For this review, take the finished solid that the model builds, in its own axes (mm). A direction names the side the tool comes from. Coordinates: 2 decimals unless noted, no trailing zeros. Write each loop counter-clockwise with the first axis right and the second up, starting at its lowest first coordinate (ties: lowest second). Pieces come first, ordered by that corner, then holes. Notation, with made-up numbers: (84, 40) -> (142, 40) arc R18 cw to (142, 72) -> close; hole circle Ø10 at (21.25, 21.5). An arc over 180 degrees is marked (long way). One line per item, written item: value. Start each with the question number.
1) Add section A-A (y = 50). State the section outline as (x, z) points, and give its area (3 significant figures).
2) For probe 1 along Y at (x, z) = (53, 51.5); probe 2 along X at (y, z) = (39, 12.5); probe 3 along Z at (x, y) = (0.95, -50), list the stretches that pass through material, from the lowest coordinate up. Write a range as from..to.
3) Add section B-B (z = 35). State the section outline as (x, y) points.
4) Add section D-D (x = 13). State the section outline as (y, z) points, and give its area (4 significant figures).
5) Add section C-C (y = 27). State the section outline as (x, z) points, and give its area (3 significant figures).
6) Mouldability with a two-part tool opening along Z and no side actions: class faces 1 (the flat face through (30, 63.5, 39)), 2 (the flat face through (35, 1, 0)), 3 (the cylindrical face through (0.7, -49.6, 3.4)) as released by +Z, released by -Z, zero draft, split by the parting line, or undercut.
7) For pin 1 Ø22.5 at (x, y) = (34, 48) entering from +Z; pin 2 Ø3 at (y, z) = (-8.5, 73.39) entering from -X, all flat-tipped, find the tip position at first contact; note any pin that passes through.
8) Machinability: for faces 4 (the cylindrical face through (0.74, -24.12, 63.17)), 5 (the flat face through (31, -62, 40)), 6 (the flat face through (1, 0, 80)), which of the approach directions +Z, -Z, +X, -X, +Y, -Y give a long, thin tool a straight path to every point of the face, cutting with its end or side? Answer none if there is none.
from build123d import *

# Parameters (mm, degrees)
PAD_DEPTH       = 80
POCKET_DEPTH    = 79.001
SKETCH002_R     = 1.65
POCKET001_DEPTH = 5


with BuildPart() as part:
    # Sketch → Pad (new body)
    with BuildSketch(Plane.XY):
        with BuildLine():
            Line((0, 63.5), (60, 63.5))
            ThreePointArc((70, 53.5), (67.071068, 60.571068), (60, 63.5))
            Line((70, 53.5), (70, -53.5))
            ThreePointArc((60, -63.5), (67.071068, -60.571068), (70, -53.5))
            Line((60, -63.5), (0, -63.5))
            Line((0, -63.5), (0, 63.5))
        make_face()
    extrude(amount=PAD_DEPTH)

    # Sketch001 → Pocket (cut, through all)
    with BuildSketch(Plane.XY.offset(1)):
        with BuildLine():
            Line((1.5, 62), (60, 62))
            ThreePointArc((68.5, 53.5), (66.010408, 59.510408), (60, 62))
            Line((68.5, 53.5), (68.5, 17))
            Line((68.5, 17), (1.5, 17))
            Line((1.5, 17), (1.5, 62))
        make_face()
        with BuildLine():
            Line((1.5, 15.5), (68.5, 15.5))
            Line((68.5, 15.5), (68.5, -53.5))
            ThreePointArc((60, -62), (66.010408, -59.510408), (68.5, -53.5))
            Line((60, -62), (1.5, -62))
            Line((1.5, -62), (1.5, 15.5))
        make_face()
    extrude(amount=POCKET_DEPTH, mode=Mode.SUBTRACT)

    # Sketch002 → Pocket001 (cut)
    with BuildSketch(Plane(origin=(0, 0, 0), x_dir=(0, -1, 0), z_dir=(-1, 0, 0))):
        with Locations((-50, 5)):
            Circle(SKETCH002_R)
        with Locations((50, 5)):
            Circle(SKETCH002_R)
        with Locations((8.5, 73.394079)):
            Circle(SKETCH002_R)
        with Locations((24.47625, 64.779078)):
            Circle(SKETCH002_R)
    extrude(amount=-POCKET001_DEPTH, mode=Mode.SUBTRACT)


solid = part.part
Numbers:
1. outline: (0, 0) -> (70, 0) -> (70, 80) -> (68.5, 80) -> (68.5, 1) -> (1.5, 1) -> (1.5, 3.35) -> (0, 3.35) -> close; (0, 6.65) -> (1.5, 6.65) -> (1.5, 80) -> (0, 80) -> close
1. area: 302 mm²
2. probe 1: -63.5..-62, 15.5..17, 62..63.5
2. probe 2: 0..1.5, 68.5..70
2. probe 3: 0..3.35, 6.65..80
3. outline: (0, -63.5) -> (60, -63.5) arc R10 ccw to (70, -53.5) -> (70, 53.5) arc R10 ccw to (60, 63.5) -> (0, 63.5) -> close; hole (1.5, -62) -> (60, -62) arc R8.5 ccw to (68.5, -53.5) -> (68.5, 15.5) -> (1.5, 15.5) -> close; hole (1.5, 17) -> (68.5, 17) -> (68.5, 53.5) arc R8.5 ccw to (60, 62) -> (1.5, 62) -> close
4. outline: (-63.5, 0) -> (63.5, 0) -> (63.5, 80) -> (62, 80) -> (62, 1) -> (17, 1) -> (17, 80) -> (15.5, 80) -> (15.5, 1) -> (-62, 1) -> (-62, 80) -> (-63.5, 80) -> close
4. area: 482.5 mm²
5. outline: (0, 0) -> (70, 0) -> (70, 80) -> (68.5, 80) -> (68.5, 1) -> (1.5, 1) -> (1.5, 80) -> (0, 80) -> close
5. area: 307 mm²
6. face 1: zero draft
6. face 2: released by -Z
6. face 3: undercut
7. pin 1: z = 1
7. pin 2: x = 68.5
8. face 4: -X
8. face 5: +Z
8. face 6: +Z, +X, -X, +Y, -Y
